Check sheet for the modelled part. Datum: model origin and axes. Units: mm. A direction names the side the tool comes from. Round coordinates to 2 decimals unless told otherwise and drop trailing zeros.
Item 1: Tool access check on faces 3 (the flat face through (34.738, 3.227, 10.898)), 4 (the flat face through (21.1, 127.67, 29.67)), 5 (the flat face through (-0.37, 125.84, -39.37)). Record the directions out of +Z, -Z, +X, -X, +Y, -Y that give a thin tool (end or side, any length) a straight path to the whole face; none if there is none.
Item 2: Release check for a two-part mould opening along Y. For faces 1 (the flat face through (-22.84, 125.84, 32.07)), 2 (the flat face through (-34.51, 127.67, -11.6)) record: +Y half, -Y half, draft (parallel to the pull), parting line (faces both ways), or undercut.
Item 3: Go/stop test with flat-tipped pins: pin 1 Ø4 at (x, y) = (44, 91) entering from -Z; pin 2 Ø1.5 at (y, z) = (113, 19.5) entering from +X; pin 3 Ø2 at (x, y) = (-9, 2) entering from -Z. Record where each tip stops, or that it passes through.
Item 4: Cross-section at A-A on z = 9.5. Count the separate pieces of the cut face and the enclosed holes in it, plus the area to 3 significant figures.
Item 5: Material ranges on line 1 (Y direction, x = 59, z = 45); line 2 (Y direction, x = 28, z = 69); line 3 (Z direction, x = -2, y = 34.5), recorded low to high.
from build123d import *

# Parameters (mm, degrees)
CREATION_EXTRUDE_DEPTH = 130.901699304
CREATION_EXTRUDE_TAPER = -26.56505118
SKETCH2_OUTSIDE_W      = 455.432
SKETCH2_OUTSIDE_H      = 443.246
CREATION_CUT_DEPTH     = 130.901699304
CREATION_CUT_TAPER     = 26.56505118
CUT_EXTRUDE_A_DEPTH    = 25.4
A_INV_DEPTH            = 25.4
CUT_EXTRUDE_B_DEPTH    = 25.4
B_INV_DEPTH            = 25.4
CUT_EXTRUDE_C_DEPTH    = 25.4
C_INV_DEPTH            = 25.4
CUT_EXTRUDE_D_DEPTH    = 25.4
D_INV_DEPTH            = 25.4
CUT_EXTRUDE_E_DEPTH    = 25.4
E_INV_DEPTH            = 25.4
CUT_EXTRUDE_F_DEPTH    = 25.4
F_INV_DEPTH            = 25.4


with BuildPart() as part:
    # Sketch1 → creation_extrude (new body)
    with BuildSketch(Plane(origin=(0, 0, 0), x_dir=(1, 0, 0), z_dir=(0, 1, 0))):
        Polygon((0, 49.999999949), (-47.552825766, 15.450849703), (-29.389262585, -40.450849677), (29.389262585, -40.450849677), (47.552825766, 15.450849703), align=None)
    extrude(amount=CREATION_EXTRUDE_DEPTH, taper=CREATION_EXTRUDE_TAPER)

    # Sketch2 outside → creation_cut (cut)
    with BuildSketch(Plane(origin=(0, 130.901699304, 0), x_dir=(1, 0, 0), z_dir=(0, 1, 0))):
        with Locations((0, 12.5)):
            Rectangle(SKETCH2_OUTSIDE_W, SKETCH2_OUTSIDE_H)
        Polygon((0, -49.999999949), (47.552825766, -15.450849703), (29.389262585, 40.450849677), (-29.389262585, 40.450849677), (-47.552825766, -15.450849703), align=None, mode=Mode.SUBTRACT)
    extrude(amount=-CREATION_CUT_DEPTH, taper=CREATION_CUT_TAPER, mode=Mode.SUBTRACT)

    # Sketch3 → Cut-Extrude A (cut)
    with BuildSketch(Plane(origin=(0, 130.901699304, 0), x_dir=(1, 0, 0), z_dir=(0, 1, 0))):
        Polygon((0, -44.999999954), (42.79754319, -13.905764733), (26.450336326, 36.40576471), (-26.450336326, 36.40576471), (-42.79754319, -13.905764733), align=None)
    extrude(amount=-CUT_EXTRUDE_A_DEPTH, mode=Mode.SUBTRACT)

    # Sketch4 → A_inv (cut)
    with BuildSketch(Plane.XZ):
        Polygon((0, -44.999999954), (42.79754319, -13.905764733), (26.450336326, 36.40576471), (-26.450336326, 36.40576471), (-42.79754319, -13.905764733), align=None)
    extrude(amount=-A_INV_DEPTH, mode=Mode.SUBTRACT)

    # Sketch5 → Cut-Extrude B (cut)
    with BuildSketch(Plane(origin=(0, 42.360679738, -84.721359466), x_dir=(-1, 0, 0), z_dir=(-9.08060963965006e-15, 0.4472135955455734, -0.8944271909771081))):
        Polygon((-42.797543189, 44.635254864), (1e-09, 13.541019643), (42.79754319, 44.635254866), (26.450336325, 94.946784308), (-26.450336327, 94.946784307), align=None)
    extrude(amount=-CUT_EXTRUDE_B_DEPTH, mode=Mode.SUBTRACT)

    # Sketch6 → B_inv (cut)
    with BuildSketch(Plane(origin=(0, -16.180339872, 32.36067974), x_dir=(1, 0, 0), z_dir=(4.012362398915141e-15, -0.44721359554557344, 0.8944271909771081))):
        Polygon((-42.797543187, 72.446784338), (-26.450336325, 22.135254895), (26.450336328, 22.135254894), (42.797543192, 72.446784336), (3e-09, 103.541019559), align=None)
    extrude(amount=-B_INV_DEPTH, mode=Mode.SUBTRACT)

    # Sketch7 → Cut-Extrude C (cut)
    with BuildSketch(Plane(origin=(80.574800989, 42.360679738, -26.180339862), x_dir=(-0.24464430830200606, -0.12861712429362887, -0.9610446387935736), z_dir=(0.8506508083303457, 0.44721359554557377, -0.2763932022429817))):
        Polygon((35.93427446, 50.325575991), (12.522250638, 97.763517638), (-39.828626118, 90.15648997), (-48.771223472, 38.017146671), (-1.947175829, 13.400288029), align=None)
    extrude(amount=-CUT_EXTRUDE_C_DEPTH, mode=Mode.SUBTRACT)

    # Sketch8 → C_inv (cut)
    with BuildSketch(Plane(origin=(-30.776835339, -16.180339872, 9.999999989), x_dir=(0.2446443083020028, 0.12861712429362696, 0.9610446387935747), z_dir=(-0.8506508083303469, -0.4472135955455736, 0.27639320224297786))):
        Polygon((-31.935023341, 77.848060657), (-22.992425992, 25.708717357), (29.358450763, 18.101689683), (52.77047459, 65.539631327), (14.889024305, 102.464919293), align=None)
    extrude(amount=-C_INV_DEPTH, mode=Mode.SUBTRACT)

    # Sketch9 → Cut-Extrude D (cut)
    with BuildSketch(Plane(origin=(49.797965648, 42.360679738, 68.541019594), x_dir=(0.8506508083603209, -0.27639320226847824, -0.44721359547279954), z_dir=(0.5257311121057348, 0.44721359554557366, 0.7236067977315217))):
        Polygon((-4.184405192, 98.473361345), (-54.495934634, 82.126154482), (-54.495934634, 29.22548183), (-4.184405192, 12.878274966), (26.90983003, 55.675818156), align=None)
    extrude(amount=-CUT_EXTRUDE_D_DEPTH, mode=Mode.SUBTRACT)

    # Sketch10 → D_inv (cut)
    with BuildSketch(Plane(origin=(-19.021130306, -16.180339872, -26.180339859), x_dir=(-0.8506508083603233, 0.27639320226847536, 0.44721359547279665), z_dir=(-0.5257311121057309, -0.44721359554557344, -0.7236067977315247))):
        Polygon((31.995934659, 98.473361351), (-18.315594783, 82.126154488), (-18.315594783, 29.225481836), (31.995934659, 12.878274972), (63.090169881, 55.675818162), align=None)
    extrude(amount=-D_INV_DEPTH, mode=Mode.SUBTRACT)

    # Sketch11 → Cut-Extrude E (cut)
    with BuildSketch(Plane(origin=(-49.797965648, 42.360679738, 68.541019594), x_dir=(0.8506508083603298, 0.2763932022684677, 0.447213595472789), z_dir=(-0.5257311121057203, 0.44721359554557355, 0.7236067977315324))):
        Polygon((4.184405192, 98.473361345), (-26.90983003, 55.675818156), (4.184405192, 12.878274966), (54.495934634, 29.22548183), (54.495934634, 82.126154482), align=None)
    extrude(amount=-CUT_EXTRUDE_E_DEPTH, mode=Mode.SUBTRACT)

    # Sketch12 → E_inv (cut)
    with BuildSketch(Plane(origin=(19.021130306, -16.180339872, -26.180339859), x_dir=(-0.8506508083603274, -0.27639320226847064, -0.44721359547279194), z_dir=(0.5257311121057243, -0.44721359554557355, -0.7236067977315294))):
        Polygon((-31.99593466, 98.473361351), (-63.090169881, 55.67581816), (-31.995934658, 12.878274972), (18.315594784, 29.225481837), (18.315594782, 82.126154489), align=None)
    extrude(amount=-E_INV_DEPTH, mode=Mode.SUBTRACT)

    # Sketch13 → Cut-Extrude F (cut)
    with BuildSketch(Plane(origin=(-80.574800989, 42.360679738, -26.180339862), x_dir=(-0.2446443083019911, 0.12861712429362016, 0.9610446387935785), z_dir=(-0.8506508083303512, 0.44721359554557344, -0.2763932022429644))):
        Polygon((-12.522250637, 97.763517637), (-35.934274461, 50.325575991), (1.947175826, 13.400288027), (48.771223471, 38.017146666), (39.828626119, 90.156489966), align=None)
    extrude(amount=-CUT_EXTRUDE_F_DEPTH, mode=Mode.SUBTRACT)

    # Sketch14 → F_inv (cut)
    with BuildSketch(Plane(origin=(30.776835339, -16.180339872, 9.999999989), x_dir=(0.2446443083019939, -0.12861712429362177, -0.9610446387935776), z_dir=(0.8506508083303502, -0.4472135955455736, 0.2763932022429676))):
        Polygon((-29.358450768, 18.101689686), (22.992425988, 25.708717353), (31.935023344, 77.848060652), (-14.889024299, 102.464919294), (-52.770474589, 65.539631333), align=None)
    extrude(amount=-F_INV_DEPTH, mode=Mode.SUBTRACT)


with BuildPart() as f_inv_kept_piece:
    # of the separate pieces the step leaves, the one the design keeps (f_inv_pieces_kept)
    add(part.part.solids().sort_by_distance((0, 0, -49.999999949))[0])


solid = f_inv_kept_piece.part
Response values:
1. face 3: -Y
1. face 4: +Y
1. face 5: -Z
2. face 1: undercut
2. face 2: draft
3. pin 1: stops at z = -61.4
3. pin 2: stops at x = 58.39
3. pin 3: stops at z = -45.65
4. separate pieces: 6
4. enclosed holes: 0
4. area: 174 mm2
5. line 1: y = 60.8 to 67.97
5. line 2: y = 58.52 to 65.82
5. line 3: z = -69.87 to -66.08
